Input: part model. Units: mm. Frame: model coordinates. A direction names the side the tool comes from. Coordinates: 2 decimals unless noted, no trailing zeros. Order: outer loops, then holes, each group sorted by start corner. A loop starts at its lowest first (then second) coordinate and runs counter-clockwise, first axis right, second up. Notation, with made-up numbers: (29, -40) - (44, -40) arc R14 cw to (44, -25) - close; hole circle Ø11 at (13, 54). An arc over 180 degrees is marked (long way). Answer as CSV lines item,"result". Start each with the question number.
Item 1: First-contact query: pin 1 (7 mm diameter, centred on x = -36.51, y = -271.46, fed in from -Z); pin 2 (10 mm diameter, centred on y = -61.5, z = 13, fed in from +X) (3 decimals); pin 3 (3 mm diameter, centred on x = -36.51, y = -7.94, fed in from +Z); pin 4 (8.5 mm diameter, centred on x = -11.11, y = -271.46, fed in from +Z) (3 decimals). Flat tips, straight axial feed; report the tip coordinate or a pass-through.
Item 2: Section A-A (y = -195.5). Output: boundary loops of the cut face in (x, z) (3 decimals), and give its area (3 significant figures).
Item 3: Material intervals for line 1 along X through (y, z) = (-124, 16) (3 decimals); line 2 along Z through (x, y) = (-38, -192.5) (3 decimals); line 3 along X through (y, z) = (-21, 48.5), sorted ascending.
Item 4: Draft query along Z for faces 3 (the cylindrical face through (-49.19, -37.27, 38.69)), 4 (the cylindrical face through (-36.85, -294.27, 1.61)), 5 (the flat face through (-26, -150, 0)). Return one class per face: +Z half, -Z half, draft (parallel to the pull), parting line (faces both ways), or undercut.
Item 5: Section C-C (z = 30.5). Output: boundary loops of the cut face in (x, y) (3 decimals), and give its area (3 significant figures).
Item 6: Section B-B (x = -23.5). Output: boundary loops of the cut face in (y, z) (3 decimals).
Item 7: Access query for faces 1 (the flat face through (-37, -304.8, 3)), 2 (the flat face through (-24, -150, 3.175)). Directions: +Z, -Z, +X, -X, +Y, -Y. A direction counts if a zero-diameter tool reaches every point of the face in a straight line with its end or side. Return the directions, or none.
from build123d import *

# Parameters (mm, degrees)
F1_DEPTH = 304.8
F2_R     = 2.6162
F3_DEPTH = 3.176
F4_R     = 2.6162
F5_DEPTH = 3.176
F6_R     = 2.6162
F7_DEPTH = 50.801


with BuildPart() as f1:
    # F0 (on Front) → F1 (new body)
    with BuildSketch(Plane.XZ):
        with BuildLine():
            Line((-50.8, 0), (0, 0))
            ThreePointArc((0, 0), (-0.929936, 2.245064), (-3.175, 3.175))
            Line((-3.175, 3.175), (-44.45, 3.175))
            ThreePointArc((-44.45, 3.175), (-46.695064, 4.104936), (-47.625, 6.35))
            Line((-47.625, 6.35), (-47.625, 47.625))
            ThreePointArc((-47.625, 47.625), (-48.554936, 49.870064), (-50.8, 50.8))
            Line((-50.8, 50.8), (-50.8, 0))
        make_face()
    extrude(amount=F1_DEPTH)

    # F2 (on face) → F3 (cut, through all)
    with BuildSketch(Plane.YZ.offset(-47.625)):
        with Locations((-14.2875, 14.2875)):
            Circle(F2_R)
        with Locations((-39.6875, 14.2875)):
            Circle(F2_R)
        with Locations((-14.2875, 39.6875)):
            Circle(F2_R)
        with Locations((-39.6875, 39.6875)):
            Circle(F2_R)
    extrude(amount=-F3_DEPTH, mode=Mode.SUBTRACT)

    # F4 (on face) → F5 (cut, through all)
    with BuildSketch(Plane.XY.offset(3.175)):
        with Locations((-36.5125, -296.8625)):
            Circle(F4_R)
        with Locations((-36.5125, -7.9375)):
            Circle(F4_R)
        with Locations((-11.1125, -7.9375)):
            Circle(F4_R)
        with Locations((-11.1125, -296.8625)):
            Circle(F4_R)
        with Locations((-11.1125, -271.4625)):
            Circle(F4_R)
        with Locations((-36.5125, -271.4625)):
            Circle(F4_R)
        with Locations((-11.1125, -33.3375)):
            Circle(F4_R)
        with Locations((-36.5125, -33.3375)):
            Circle(F4_R)
    extrude(amount=-F5_DEPTH, mode=Mode.SUBTRACT)

    # F6 (on face) → F7 (cut, through all)
    with BuildSketch(Plane(origin=(-50.8, 0, 0), x_dir=(0, -1, 0), z_dir=(-1, 0, 0))):
        with Locations((166.3319, 42.8625)):
            Circle(F6_R)
    extrude(amount=-F7_DEPTH, mode=Mode.SUBTRACT)


solid = f1.part
Determined:
1,pin 1,"stops at z = 0"
1,pin 2,"stops at x = -47.625"
1,pin 3,"passes through"
1,pin 4,"stops at z = 3.175"
2,outline,"(-50.8, 0) - (0, 0) arc R3.175 ccw to (-3.175, 3.175) - (-44.45, 3.175) arc R3.175 cw to (-47.625, 6.35) - (-47.625, 47.625) arc R3.175 ccw to (-50.8, 50.8) - close"
2,area,"310 mm^2"
3,line 1,"x = -50.8 to -47.625"
3,line 2,"z = 0 to 3.175"
3,line 3,"x = -50.8 to -47.75"
4,face 3,"undercut"
4,face 4,"draft"
4,face 5,"-Z half"
5,outline,"(-50.8, -304.8) - (-47.625, -304.8) - (-47.625, 0) - (-50.8, 0) - close"
5,area,"968 mm^2"
6,outline,"(-304.8, 0) - (0, 0) - (0, 3.175) - (-304.8, 3.175) - close"
7,face 1,"+Z, -Z, +X, -X, -Y"
7,face 2,"+Z, +X, +Y, -Y"
